Part model, mm, in its own coordinate system. A direction names the side the tool comes from. Round coordinates to 2 decimals unless told otherwise and drop trailing zeros. Loops run counter-clockwise (first coordinate to the right, second up) from the corner with the lowest first, then second, coordinate; pieces in that order, holes last.
1) Band-saw the part on C-C, the plane z = 3.75. Write the cut outline in (x, y), then the cut area to 3 significant figures.
2) Band-saw the part on A-A, the plane x = -3.5. Write the cut outline in (y, z), then the cut area to 3 significant figures.
3) 3-axis set-ups, long thin cutter, end or side, ignore diameter. For faces 1 (the cylindrical face through (20.53, 0.9, 0.89)), 2 (the cylindrical face through (25.275, -5.163, 3.698)): which of +Z, -Z, +X, -X, +Y, -Y reach the whole face in a straight line?
4) Band-saw the part on D-D, the plane x = 16.5. Write the cut outline in (y, z).
5) Drop flat-ended pins along their axis: P1, Ø1.5, axis at x = -1.5, z = 1.5, coming from the -Y side; P2, Ø10, axis at x = 15.5, y = 6.5, coming from the -Z side; P3, Ø3, axis at y = -0.5, z = 2.5, coming from the +X side. Give the stop position or say it passes through.
6) Mould opens along Y. For faces 3 (the flat face through (5, -10, 4)), 4 (the cylindrical face through (6.466, -2.681, 3.698)), 5 (the cylindrical face through (12.497, 9.844, 3.698)) say: +Y half, -Y half, draft (parallel to the pull), parting line (faces both ways), or undercut.
7) Probe line 1 (Y direction, x = 0, z = 5.75); line 2 (Y direction, x = -3, z = 4.75); line 3 (X direction, y = 0.5, z = 0.5). List the from-to ranges inside material, lowest first.
8) Band-saw the part on B-B, the plane y = 0. Write the cut outline in (x, z), then the cut area to 3 significant figures.
from build123d import *

# Parameters (mm, degrees)
SKETCH1_R           = 7
BOSS_EXTRUDE1_DEPTH = 7.5
SKETCH2_R           = 3
CUT_EXTRUDE1_DEPTH  = 10


with BuildPart() as part:
    # Sketch1 → Boss-Extrude1 (new body)
    with BuildSketch(Plane.XY):
        with BuildLine():
            Line((25.460451105, -4.582574037), (25.460451105, 4.582574037))
            ThreePointArc((25.460451105, 4.582574037), (25.279603149, 5.156150473), (24.802471248, 5.522266658))
            Line((24.802471248, 5.522266658), (14.156931626, 9.396926208))
            ThreePointArc((14.156931626, 9.396926208), (12.47321197, 9.84807753), (10.736730193, 10))
            Line((10.736730193, 10), (0, 10))
            ThreePointArc((0, 10), (-10, 0), (0, -10))
            Line((0, -10), (10.736730193, -10))
            ThreePointArc((10.736730193, -10), (12.47321197, -9.84807753), (14.156931626, -9.396926208))
            Line((14.156931626, -9.396926208), (24.802471248, -5.522266658))
            ThreePointArc((24.802471248, -5.522266658), (25.279603149, -5.156150473), (25.460451105, -4.582574037))
        make_face()
        Circle(SKETCH1_R, mode=Mode.SUBTRACT)
    extrude(amount=BOSS_EXTRUDE1_DEPTH)

    # Sketch2 → Cut-Extrude1 (cut)
    with BuildSketch(Plane(origin=(25.460451105, 0, 0), x_dir=(0, 0, -1), z_dir=(1, 0, 0))):
        with Locations((-3.75, 0)):
            Circle(SKETCH2_R)
    extrude(amount=-CUT_EXTRUDE1_DEPTH, mode=Mode.SUBTRACT)


solid = part.part
Reported:
1. outline: (0, -10) - (10.74, -10) arc R10 ccw to (14.16, -9.4) - (24.8, -5.52) arc R1 ccw to (25.46, -4.58) - (25.46, -3) - (15.46, -3) - (15.46, 3) - (25.46, 3) - (25.46, 4.58) arc R1 ccw to (24.8, 5.52) - (14.16, 9.4) arc R10 ccw to (10.74, 10) - (0, 10) arc R10 ccw to start; hole circle Ø14 at (0, 0)
1. area: 391 mm2
2. outline: (-9.37, 0) - (-6.06, 0) - (-6.06, 7.5) - (-9.37, 7.5) - close; (6.06, 0) - (9.37, 0) - (9.37, 7.5) - (6.06, 7.5) - close
2. area: 49.6 mm2
3. face 1: +X
3. face 2: +Z, -Z, +X, -Y
4. outline: (-8.54, 0) - (8.54, 0) - (8.54, 7.5) - (-8.54, 7.5) - close; hole circle Ø6 at (0, 3.75)
5. P1: stops at y = -9.97
5. P2: stops at z = 0
5. P3: stops at x = 15.46
6. face 3: -Y half
6. face 4: undercut
6. face 5: +Y half
7. line 1: y = -10 to -7, 7 to 10
7. line 2: y = -9.54 to -6.32, 6.32 to 9.54
7. line 3: x = -9.99 to -6.98, 6.98 to 25.46
8. outline: (-10, 0) - (-7, 0) - (-7, 7.5) - (-10, 7.5) - close; (7, 0) - (25.46, 0) - (25.46, 0.75) - (15.46, 0.75) - (15.46, 6.75) - (25.46, 6.75) - (25.46, 7.5) - (7, 7.5) - close
8. area: 101 mm2
